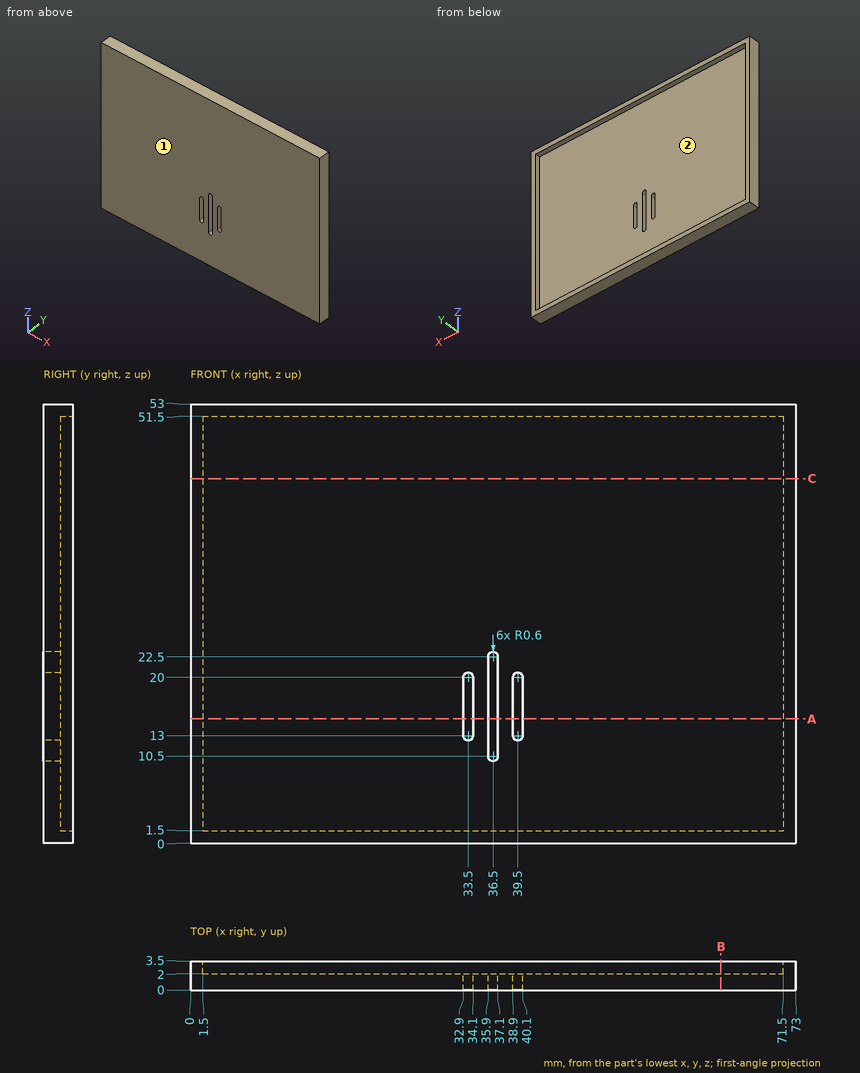
Here's the drawing with two shaded views (mm, measured from the low corner). I have some questions. Coordinates: 2 decimals unless noted, no trailing zeros. Order: outer loops, then holes, each group sorted by start corner. A loop starts at its lowest first (then second) coordinate and runs counter-clockwise, first axis right, second up. Notation, with made-up numbers: M 70,-6 L 118,-6 A24 cw 118,4 Z; hole C -17.75,20.25 d6. An arc over 180 degrees is marked long. Write item = value, one per line.
(1) Suppose I cut it at B-B on x = 64. Please give me the cut outline in (y, z), plus the area to 4 significant figures.
Results are:
outline = M 0,0 L 3.5,0 L 3.5,1.5 L 2,1.5 L 2,51.5 L 3.5,51.5 L 3.5,53 L 0,53 Z
area = 110.5 mm2
(2) Suppose I cut it at A-A on z = 15. Please give me the cut outline in (x, y), plus the area to 3 significant figures.
Results are:
outline = M 0,0 L 32.9,0 L 32.9,2 L 1.5,2 L 1.5,3.5 L 0,3.5 Z; M 34.1,0 L 35.9,0 L 35.9,2 L 34.1,2 Z; M 37.1,0 L 38.9,0 L 38.9,2 L 37.1,2 Z; M 40.1,0 L 73,0 L 73,3.5 L 71.5,3.5 L 71.5,2 L 40.1,2 Z
area = 143 mm2
(3) Suppose I cut it at C-C on z = 44. Please give me the cut outline in (x, y).
Results are:
outline = M 0,0 L 73,0 L 73,3.5 L 71.5,3.5 L 71.5,2 L 1.5,2 L 1.5,3.5 L 0,3.5 Z
(4) For pin 1 Ø2 at (x, z) = (65, 45) entering from +Y, with a flat end and sliding along its axis, tell me the tip position at first contact or that it passes through.
Results are:
pin_1 = 2
(5) I need wall thicknesses on line 1 along X through (y, z) = (0.3, 14); line 2 along X through (y, z) = (1.1, 22); line 3 along X through (y, z) = (3.1, 29). Which ranges of each line are inside material? Lowest first, please. Write a range as [from, to].
Results are:
line_1 = [0, 32.9], [34.1, 35.9], [37.1, 38.9], [40.1, 73]
line_2 = [0, 35.9], [37.1, 73]
line_3 = [0, 1.5], [71.5, 73]
(6) If we mould it in two halves opening along Z, with no side actions, what happens to the marked faces 1 and 2? For each: pulls with the +Z half, pulls with the -Z half, needs draft (parallel to the pull), parting line crosses it, or undercut.
Results are:
face_1 = needs draft
face_2 = undercut
